from build123d import *

# Parameters (mm, degrees)
SKETCH1_W           = 15.8
SKETCH1_H           = 15.8
SKETCH1_W_2         = 13.8
SKETCH1_H_2         = 13.8
BOSS_EXTRUDE1_DEPTH = 600
SKETCH3_R           = 1.7
CUT_EXTRUDE2_DEPTH  = 601.25998534


with BuildPart() as part:
    # Sketch1 → Boss-Extrude1 (new body)
    with BuildSketch(Plane(origin=(0, 0, 0), x_dir=(1, 0, 0), z_dir=(0, 1, 0))):
        Rectangle(SKETCH1_W, SKETCH1_H)
        Rectangle(SKETCH1_W_2, SKETCH1_H_2, mode=Mode.SUBTRACT)
    extrude(amount=BOSS_EXTRUDE1_DEPTH)

    # Sketch3 → Cut-Extrude2 (cut, through all)
    with BuildSketch(Plane.XY.offset(7.9)):
        with Locations((0, 580)):
            Circle(SKETCH3_R)
        with Locations((0, 20)):
            Circle(SKETCH3_R)
    extrude(amount=-CUT_EXTRUDE2_DEPTH, mode=Mode.SUBTRACT)


solid = part.part
CAD build for the part. Positions are in the model's coordinates, mm. A direction names the side the tool comes from. Give positions to 0.01 mm unless a question says otherwise; leave off trailing zeros. Write each loop counter-clockwise with the first axis right and the second up, starting at its lowest first coordinate (ties: lowest second). Pieces come first, ordered by that corner, then holes. Notation, with made-up numbers: (-2, 8) - (12, 8) arc R21 cw to (12, 15) - close; hole circle Ø8 at (-5.75, 86). An arc over 180 degrees is marked (long way). Put each result on its own line as item: value.
(1) Tool access for faces 5 (the flat face through (0, 296, -6.9)), 6 (the flat face through (0, 296, -7.9)): list every direction of +Z, -Z, +X, -X, +Y, -Y with a clear straight run to the whole face (end or side of a thin tool).
Working result:
face 5: +Y, -Y
face 6: -Z, +X, -X, +Y, -Y
(2) Saw through at C-C (y = 200). List the corners of the cut face in (x, z), then the cut area to 3 significant figures.
Working result:
outline: (-7.9, -7.9) - (7.9, -7.9) - (7.9, 7.9) - (-7.9, 7.9) - close; hole (-6.9, -6.9) - (6.9, -6.9) - (6.9, 6.9) - (-6.9, 6.9) - close
area: 59.2 mm^2
(3) Saw through at B-B (x = 4.5). List the corners of the cut face in (y, z).
Working result:
outline: (0, -7.9) - (600, -7.9) - (600, -6.9) - (0, -6.9) - close; (0, 6.9) - (600, 6.9) - (600, 7.9) - (0, 7.9) - close
(4) Pull direction Z, two halves, no side cores. Call faces 1 (the flat face through (7.9, 296, 0)), 2 (the flat face through (6.9, 296, 0)), 3 (the flat face through (0, 296, 7.9)), 4 (the flat face through (-6.9, 296, 0)): released by +Z, released by -Z, zero draft, split by the parting line, or undercut.
Working result:
face 1: zero draft
face 2: undercut
face 3: released by +Z
face 4: undercut
(5) Wall check: L1, parallel to Y at x = 0, z = -7.6; L2, parallel to X at y = 580, z = -7.45; L3, parallel to X at y = 557, z = -5.5. Give the ranges that are in metal, low to high.
Working result:
L1: 0 to 18.3, 21.7 to 578.3, 581.7 to 600
L2: -7.9 to -1.7, 1.7 to 7.9
L3: -7.9 to -6.9, 6.9 to 7.9
(6) Saw through at A-A (z = 0.5). List the corners of the cut face in (x, y).
Working result:
outline: (-7.9, 0) - (-6.9, 0) - (-6.9, 600) - (-7.9, 600) - close; (6.9, 0) - (7.9, 0) - (7.9, 600) - (6.9, 600) - close
